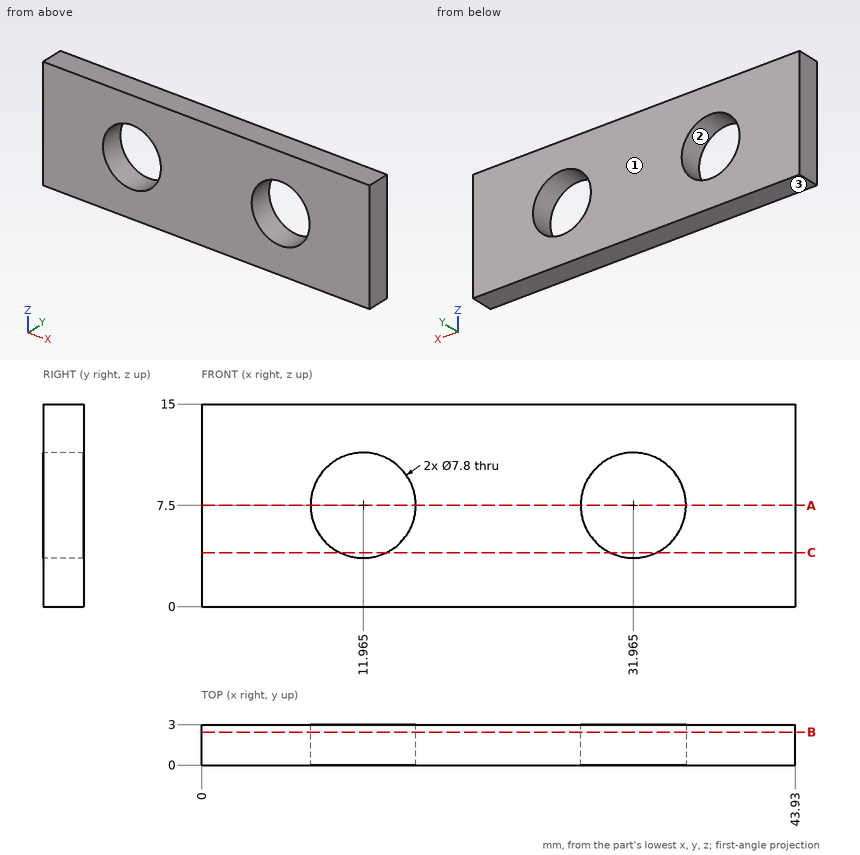
Could you check a few things on this drawing? It's one solid part, dimensions in mm from its lowest x, y, z. Give positions to 0.01 mm unless a question says otherwise; leave off trailing zeros. Write each loop counter-clockwise with the first axis right and the second up, starting at its lowest first coordinate (ties: lowest second). Pieces come first, ordered by that corner, then holes. Notation, with made-up numbers: (51, 73.5) -> (87, 73.5) arc R19 ccw to (87, 103.5) -> close; hole circle Ø11 at (70.25, 43). An arc over 180 degrees is marked (long way). Answer as a JSON object with one key per item and string values.
Q1. Suppose I cut it at B-B on y = 2.45. Write out the boundary of the cut face in (x, z) (3 decimals), then the cut area to 3 significant figures.
Taken from the geometry:
{"outline": "(0, 0) -> (43.93, 0) -> (43.93, 15) -> (0, 15) -> close; hole circle Ø7.8 at (11.965, 7.5); hole circle Ø7.8 at (31.965, 7.5)", "area": "563 mm²"}
Q2. Suppose I cut it at C-C on z = 4. Write out the boundary of the cut face in (x, y), then the cut area to 3 significant figures.
Taken from the geometry:
{"outline": "(0, 0) -> (10.24, 0) -> (10.24, 3) -> (0, 3) -> close; (13.69, 0) -> (30.24, 0) -> (30.24, 3) -> (13.69, 3) -> close; (33.69, 0) -> (43.93, 0) -> (43.93, 3) -> (33.69, 3) -> close", "area": "111 mm²"}
Q3. Please list where these lines run through material, in increasing order: L1, parallel to X at y = 2.4, z = 4.75; L2, parallel to Z at x = 35, y = 1.65; L3, parallel to X at y = 0.55, z = 6.75.
Taken from the geometry:
{"L1": "x = 0 to 9.2, 14.73 to 29.2, 34.73 to 43.93", "L2": "z = 0 to 5.05, 9.95 to 15", "L3": "x = 0 to 8.14, 15.79 to 28.14, 35.79 to 43.93"}
Q4. We'd pull the mould along Z, two halves only. Please class the marked faces 1, 2 and 3: released by +Z, released by -Z, zero draft, split by the parting line, or undercut.
Taken from the geometry:
{"face 1": "zero draft", "face 2": "undercut", "face 3": "released by -Z"}
Q5. Suppose I cut it at A-A on z = 7.5. Write out the boundary of the cut face in (x, y) (3 decimals), then the cut area to 3 significant figures.
Taken from the geometry:
{"outline": "(0, 0) -> (8.065, 0) -> (8.065, 3) -> (0, 3) -> close; (15.865, 0) -> (28.065, 0) -> (28.065, 3) -> (15.865, 3) -> close; (35.865, 0) -> (43.93, 0) -> (43.93, 3) -> (35.865, 3) -> close", "area": "85.0 mm²"}
